For this review, take the finished solid that the model builds, in its own axes (mm). A direction names the side the tool comes from. Round coordinates to 2 decimals unless told otherwise and drop trailing zeros. Write each loop counter-clockwise with the first axis right and the second up, starting at its lowest first coordinate (ties: lowest second). Pieces come first, ordered by that corner, then holes.
from build123d import *

# Parameters (mm, degrees)
F1_DEPTH = 7
F2_W     = 29
F2_H     = 8
F3_DEPTH = 5
F4_W     = 16.5
F4_H     = 7
F4_R     = 3
F5_DEPTH = 2
F0_R     = 1.5
F6_DEPTH = 1
F7_DEPTH = 3


with BuildPart() as f1:
    # F0 (on Front) → F1 (new body)
    with BuildSketch(Plane.XZ):
        Polygon((15, 3.5), (15, 6.5), (-15, 6.5), (-15, 3.5), (-15, -3.5), (-15, -6.5), (15, -6.5), (15, -3.5), align=None)
    extrude(amount=F1_DEPTH)

    # F2 (on face) → F3 (join)
    with BuildSketch(Plane.XZ.offset(7)):
        Rectangle(F2_W, F2_H)
    extrude(amount=F3_DEPTH)

    # F4 (on face) → F5 (join)
    with BuildSketch(Plane.XZ.offset(12)):
        with BuildLine():
            Line((-6.5, 3.5), (-14, 3.5))
            Line((-14, 3.5), (-14, 0))
            Line((-14, 0), (-13.25, 0))
            ThreePointArc((-13.25, 0), (-10.25, 3), (-7.25, 0))
            Line((-7.25, 0), (-6.5, 0))
            Line((-6.5, 0), (-6.5, 3.5))
        make_face()
        with BuildLine():
            Line((-13.25, 0), (-14, 0))
            Line((-14, 0), (-14, -3.5))
            Line((-14, -3.5), (-6.5, -3.5))
            Line((-6.5, -3.5), (-6.5, 0))
            Line((-6.5, 0), (-7.25, 0))
            ThreePointArc((-7.25, 0), (-10.25, -3), (-13.25, 0))
        make_face()
        with Locations((5.75, 0)):
            Rectangle(F4_W, F4_H)
        with Locations((9.739062, 0)):
            Circle(F4_R, mode=Mode.SUBTRACT)
    extrude(amount=F5_DEPTH)

    # F0 (on Front) → F6 (join)
    with BuildSketch(Plane.XZ):
        with BuildLine():
            Line((-15, -3.5), (-15, 3.5))
            Line((-15, 3.5), (-18.635049, 3.5))
            ThreePointArc((-18.635049, 3.5), (-16.160176, 2.474874), (-15.135049, 0))
            ThreePointArc((-15.135049, 0), (-16.160176, -2.474874), (-18.635049, -3.5))
            Line((-18.635049, -3.5), (-15, -3.5))
        make_face()
        with BuildLine():
            Line((18.635049, 3.5), (15, 3.5))
            Line((15, 3.5), (15, -3.5))
            Line((15, -3.5), (18.635049, -3.5))
            ThreePointArc((18.635049, -3.5), (15.135049, 0), (18.635049, 3.5))
        make_face()
        with BuildLine():
            ThreePointArc((-15.135049, 0), (-16.160176, 2.474874), (-18.635049, 3.5))
            ThreePointArc((-18.635049, 3.5), (-22.135049, 0), (-18.635049, -3.5))
            ThreePointArc((-18.635049, -3.5), (-16.160176, -2.474874), (-15.135049, 0))
        make_face()
        with Locations((-18.635049, 0)):
            Circle(F0_R, mode=Mode.SUBTRACT)
        with BuildLine():
            ThreePointArc((22.135049, 0), (21.109923, 2.474874), (18.635049, 3.5))
            ThreePointArc((18.635049, 3.5), (15.135049, 0), (18.635049, -3.5))
            ThreePointArc((18.635049, -3.5), (21.109923, -2.474874), (22.135049, 0))
        make_face()
        with Locations((18.635049, 0)):
            Circle(F0_R, mode=Mode.SUBTRACT)
    extrude(amount=F6_DEPTH)

    # F0 (on Front) → F7 (join)
    with BuildSketch(Plane.XZ):
        with BuildLine():
            Line((-15, -3.5), (-15, 3.5))
            Line((-15, 3.5), (-18.635049, 3.5))
            ThreePointArc((-18.635049, 3.5), (-16.160176, 2.474874), (-15.135049, 0))
            ThreePointArc((-15.135049, 0), (-16.160176, -2.474874), (-18.635049, -3.5))
            Line((-18.635049, -3.5), (-15, -3.5))
        make_face()
        with BuildLine():
            Line((18.635049, 3.5), (15, 3.5))
            Line((15, 3.5), (15, -3.5))
            Line((15, -3.5), (18.635049, -3.5))
            ThreePointArc((18.635049, -3.5), (15.135049, 0), (18.635049, 3.5))
        make_face()
    extrude(amount=F7_DEPTH)


solid = f1.part
(1) We need section C-C, the plane x = -18. Give the boundary of the cut face in (y, z), and give its area (3 significant figures).
Geometry check:
outline: (-3, -3.5) - (0, -3.5) - (0, -1.36) - (-1, -1.36) - (-1, -3.44) - (-3, -3.44) - close; (-3, 3.44) - (-1, 3.44) - (-1, 1.36) - (0, 1.36) - (0, 3.5) - (-3, 3.5) - close
area: 4.51 mm2
(2) We need section A-A, the plane y = -13. Give the boundary of the cut face in (x, z).
Geometry check:
outline: (-14, -3.5) - (-6.5, -3.5) - (-6.5, 3.5) - (-14, 3.5) - close; (-2.5, -3.5) - (14, -3.5) - (14, 3.5) - (-2.5, 3.5) - close; hole circle Ø6 at (-10.25, 0); hole circle Ø6 at (9.74, 0)
(3) For line 1 along Z through (x, y) = (-10.25, -13.05); line 2 along Z through (x, y) = (1, -11.75); line 3 along Y through (x, z) = (-16, -2), list the stretches that pass through material, from the lowest coordinate up.
Geometry check:
line 1: z = -3.5 to -3, 3 to 3.5
line 2: z = -4 to 4
line 3: y = -1 to 0
(4) For faces 4 (the face through (-14, -13, 0)), 5 (the face through (-6.5, -13, 0)), 6 (the face through (7.36, -12.99, -1.83)), list the 3-axis set-ups (+Z, -Z, +X, -X, +Y, -Y) from which the entire face can be reached by the end or side of a thin tool; tool diameter is ignored.
Geometry check:
face 4: +Z, -Z, -X, -Y
face 5: +Z, -Z, -Y
face 6: -Y
(5) For pin 1 Ø4 at (x, z) = (12, 3.5) entering from +Y; pin 2 Ø5 at (y, z) = (-2, -3.5) entering from -X; pin 3 Ø1 at (y, z) = (-13, -1.5) entering from +X; pin 4 Ø2.5 at (x, y) = (16.5, -1) entering from +Z, all flat-tipped, find the tip position at first contact; note any pin that passes through.
Geometry check:
pin 1: stops at y = 0
pin 2: stops at x = -21.92
pin 3: stops at x = 14
pin 4: stops at z = 3.5
(6) We need section B-B, the plane x = -10.25. Give the boundary of the cut face in (y, z).
Geometry check:
outline: (-14, -3.5) - (-12, -3.5) - (-12, -4) - (-7, -4) - (-7, -6.5) - (0, -6.5) - (0, 6.5) - (-7, 6.5) - (-7, 4) - (-12, 4) - (-12, 3.5) - (-14, 3.5) - (-14, 3) - (-12, 3) - (-12, -3) - (-14, -3) - close
(7) Mouldability with a two-part tool opening along Z and no side actions: class faces 1 (the face through (-10, -13, -3.5)), 2 (the face through (4, -14, 0)), 3 (the face through (15.136, -1.986, -0.077)) as pulls with the +Z half, pulls with the -Z half, needs draft (parallel to the pull), parting line crosses it, or undercut.
Geometry check:
face 1: pulls with the -Z half
face 2: needs draft
face 3: undercut
